from build123d import *

# Parameters (mm, degrees)
RESSALTO_EXTRUS_O1_DEPTH = 2.5
ESBO_O2_R                = 1.55
ESBO_O2_W                = 20.114167529
ESBO_O2_H                = 18
CORTE_EXTRUS_O1_DEPTH    = 3.5


with BuildPart() as part:
    # Esboço1 → Ressalto-extrusão1 (new body)
    with BuildSketch(Plane.XY):
        with BuildLine():
            Line((-82.25, 64.75), (82.25, 64.75))
            ThreePointArc((82.25, 64.75), (84.371320344, 63.871320344), (85.25, 61.75))
            Line((85.25, 61.75), (85.25, -61.75))
            ThreePointArc((85.25, -61.75), (84.371320344, -63.871320344), (82.25, -64.75))
            Line((82.25, -64.75), (-82.25, -64.75))
            ThreePointArc((-82.25, -64.75), (-84.371320344, -63.871320344), (-85.25, -61.75))
            Line((-85.25, -61.75), (-85.25, 61.75))
            ThreePointArc((-85.25, 61.75), (-84.371320344, 63.871320344), (-82.25, 64.75))
        make_face()
    extrude(amount=RESSALTO_EXTRUS_O1_DEPTH)

    # Esboço2 → Corte-extrusão1 (cut, through all)
    with BuildSketch(Plane.XY.offset(2.5)):
        with Locations((0, -57.75)):
            Circle(ESBO_O2_R)
        with Locations((-40, 57.75)):
            Circle(ESBO_O2_R)
        with Locations((40, 57.75)):
            Circle(ESBO_O2_R)
        with BuildLine():
            Line((8, 56.65), (8, 64.75))
            Line((8, 64.75), (-8, 64.75))
            Line((-8, 64.75), (-8, 56.65))
            ThreePointArc((-8, 56.65), (0, 48.65), (8, 56.65))
        make_face()
        with Locations((-70.307083765, 55.75)):
            Rectangle(ESBO_O2_W, ESBO_O2_H)
        with BuildLine():
            Line((65.25, 64.75), (75.25, 64.75))
            Line((75.25, 64.75), (75.25, 59.75))
            ThreePointArc((75.25, 59.75), (70.25, 54.75), (65.25, 59.75))
            Line((65.25, 59.75), (65.25, 64.75))
        make_face()
    extrude(amount=-CORTE_EXTRUS_O1_DEPTH, mode=Mode.SUBTRACT)


solid = part.part
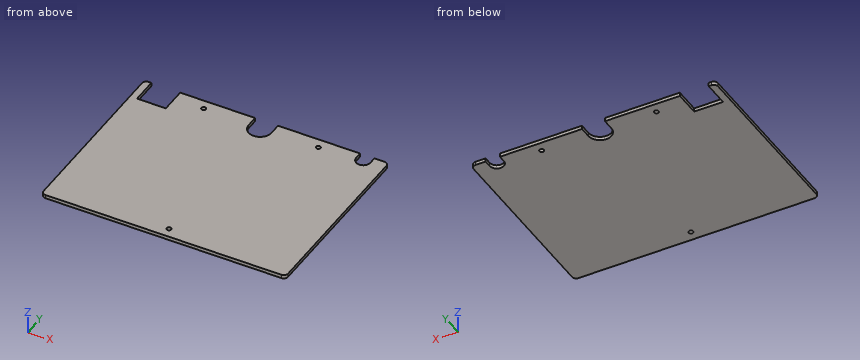
Can you work these out from the model? Positions are in its coordinate system, mm. Give positions to 0.01 mm unless a question says otherwise; leave off trailing zeros. Loops run counter-clockwise (first coordinate to the right, second up) from the corner with the lowest first, then second, coordinate; pieces in that order, holes last. Notation, with made-up numbers: (15, 54.25) -> (42, 54.25) arc R34 ccw to (42, 84.25) -> close; hole circle Ø2 at (20, -9.75). An arc over 180 degrees is marked (long way). Use one line per item in the form item = value.
1) I need wall thicknesses on line 1 along Y through (x, z) = (0, 0.85); line 2 along X through (y, z) = (47, 1.6); line 3 along Y through (x, z) = (-40, 0.65). Which ranges of each line are inside material? Lowest first, please.
Answers:
line_1 = -64.75 to -59.3, -56.2 to 48.65
line_2 = -85.25 to -80.36, -60.25 to 85.25
line_3 = -64.75 to 56.2, 59.3 to 64.75
2) Will these pins go through, and if not, where does the flat tip stop? pin 1 (0.8 mm diameter, centred on x = -74, z = 1.5, fed in from +Y); pin 2 (0.8 mm diameter, centred on y = 63, z = 1, fed in from -X); pin 3 (1.9 mm diameter, centred on x = 40, y = 57.75, fed in from +Z).
Answers:
pin_1 = 46.75
pin_2 = -85.13
pin_3 = through
3) If we section it at A-A (z = 1.25): Please give me the cut outline in (x, y), plus the area to 3 significant figures.
Answers:
outline = (-85.25, -61.75) arc R3 ccw to (-82.25, -64.75) -> (82.25, -64.75) arc R3 ccw to (85.25, -61.75) -> (85.25, 61.75) arc R3 ccw to (82.25, 64.75) -> (75.25, 64.75) -> (75.25, 59.75) arc R5 cw to (65.25, 59.75) -> (65.25, 64.75) -> (8, 64.75) -> (8, 56.65) arc R8 cw to (-8, 56.65) -> (-8, 64.75) -> (-60.25, 64.75) -> (-60.25, 46.75) -> (-80.36, 46.75) -> (-80.36, 64.75) -> (-82.25, 64.75) arc R3 ccw to (-85.25, 61.75) -> close; hole circle Ø3.1 at (-40, 57.75); hole circle Ø3.1 at (0, -57.75); hole circle Ø3.1 at (40, 57.75)
area = 21,400 mm²
